```python
from build123d import *

# Parameters (mm, degrees)
F1_DEPTH = 38.1
F3_DEPTH = 152.401


with BuildPart() as f1:
    # F0 (on Front) → F1 (new body, symmetric)
    with BuildSketch(Plane.XZ):
        Polygon((-76.2, -25.4), (76.2, -25.4), (76.2, 12.7), (6.35, 12.7), (0, 25.4), (-25.4, 25.4), (-25.4, 12.7), (-12.7, 12.7), (-12.7, 0), (-63.5, 0), (-63.5, 12.7), (-50.8, 12.7), (-50.8, 25.4), (-76.2, 25.4), align=None)
    extrude(amount=F1_DEPTH, both=True)

    # F2 (on face) → F3 (cut, through all)
    with BuildSketch(Plane.YZ.offset(76.2)):
        Polygon((25.389396, -12.7), (-25.4, -12.7), (-12.7, -25.4), (12.7, -25.4), align=None)
    extrude(amount=-F3_DEPTH, mode=Mode.SUBTRACT)


solid = f1.part
```
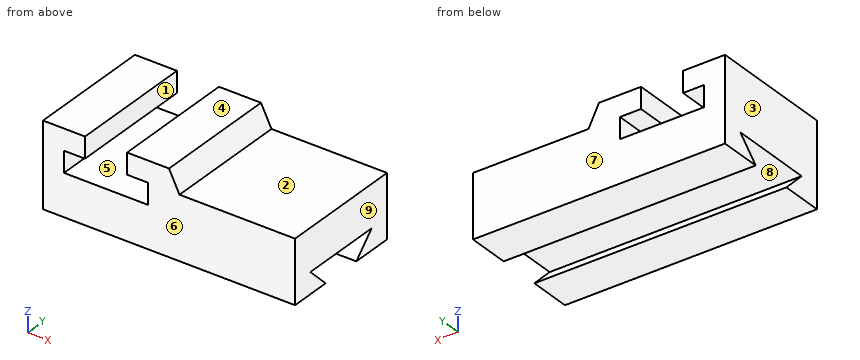
Model file for the job. Use its own axes, mm. Face numbers are marked on the shaded views. A direction names the side the tool comes from. Round coordinates to 2 decimals unless told otherwise and drop trailing zeros. Loops run counter-clockwise (first coordinate to the right, second up) from the corner with the lowest first, then second, coordinate; pieces in that order, holes last. Notation, with made-up numbers: M 42.5,-1.5 L 85.5,-1.5 A9 ccw 85.5,11.5 Z; hole C -23.5,7 d5. An arc over 180 degrees is marked long. Put each result on its own line as item: value. Start each with the question number.
Item 1: Drop flat-ended pins along their axis: P1, Ø6.5, axis at x = -57, y = -4.5, coming from the -Z side; P2, Ø10, axis at y = -10.5, z = 21.5, coming from the +X side; P3, Ø3, axis at x = 56, y = 14, coming from the +Z side. Give the stop position or say it passes through.
Item 2: 3-axis set-ups, long thin cutter, end or side, ignore diameter. For the marked faces 1, 2, 3, 4 and 5: which of +Z, -Z, +X, -X, +Y, -Y reach the whole face in a straight line?
Item 3: Drill centre lines: line 1 along X through (y, z) = (7.5, 9); line 2 along Y through (x, z) = (-29.5, -17); line 3 along X through (y, z) = (-19, 14.5). Where is each one in solid material? Low to high.
Item 4: Mould opens along Y. For the marked faces 6, 7, 8 and 9 say: released by +Y, released by -Y, zero draft, split by the parting line, or undercut.
Item 5: Cut at D-D (x = -37). List the corners of the cut face in (y, z), then the cut area to 3 significant figures.
Item 6: Cut at B-B (x = -58). List the corners of the cut face in (y, z), then the cut area to 3 significant figures.
Item 7: Cut at A-A (z = 7.5). List the corners of the cut face in (x, y).
Item 8: Cut at C-C (y = 1). List the corners of the cut face in (x, z).
Answer block:
1. P1: z = -12.7
1. P2: x = 4.45
1. P3: z = 12.7
2. face 1: +Z, +Y, -Y
2. face 2: +Z, +X, +Y, -Y
2. face 3: +Z, -Z, -X, +Y, -Y
2. face 4: +Z, +X, -X, +Y, -Y
2. face 5: +Y, -Y
3. line 1: -76.2 to -63.5, -12.7 to 76.2
3. line 2: -38.1 to -21.1, 21.09 to 38.1
3. line 3: -76.2 to -50.8, -25.4 to 5.45
4. face 6: released by -Y
4. face 7: released by +Y
4. face 8: undercut
4. face 9: zero draft
5. outline: M -38.1,-25.4 L -12.7,-25.4 L -25.4,-12.7 L 25.39,-12.7 L 12.7,-25.4 L 38.1,-25.4 L 38.1,0 L -38.1,0 Z
5. area: 1,450 mm2
6. outline: M -38.1,-25.4 L -12.7,-25.4 L -25.4,-12.7 L 25.39,-12.7 L 12.7,-25.4 L 38.1,-25.4 L 38.1,0 L -38.1,0 Z; M -38.1,12.7 L 38.1,12.7 L 38.1,25.4 L -38.1,25.4 Z
6. area: 2,420 mm2
7. outline: M -76.2,-38.1 L -63.5,-38.1 L -63.5,38.1 L -76.2,38.1 Z; M -12.7,-38.1 L 76.2,-38.1 L 76.2,38.1 L -12.7,38.1 Z
8. outline: M -76.2,-12.7 L 76.2,-12.7 L 76.2,12.7 L 6.35,12.7 L 0,25.4 L -25.4,25.4 L -25.4,12.7 L -12.7,12.7 L -12.7,0 L -63.5,0 L -63.5,12.7 L -50.8,12.7 L -50.8,25.4 L -76.2,25.4 Z
